The listing builds one solid part. Answer for the finished solid, in the listing's coordinates (mm). A direction names the side the tool comes from. Give positions to 0.01 mm unless a question says otherwise; leave off trailing zeros. Loops run counter-clockwise (first coordinate to the right, second up) from the corner with the lowest first, then second, coordinate; pieces in that order, holes last. Notation, with made-up numbers: (13, 59.5) - (20, 59.5) arc R24 cw to (20, 89.5) - close; hole circle Ø3 at (-10.75, -30.75). An arc over 180 degrees is marked (long way). Answer as CSV lines item,"result". Start each with the question number.
1) A cutting plane is placed at C-C (z = -11.5). Determine the outline of the cut face in (x, y), and give its area (3 significant figures).
2) A cutting plane is placed at D-D (x = 28). Determine the outline of the cut face in (y, z).
3) For a pull along Z with two mould halves and no side action, classify faces 3 (the face through (15.02, -0.02, 47.69)), 4 (the face through (18.377, 1.327, -36.344)), 5 (the face through (-1, -1.5, -1)) as pulls with the +Z half, pulls with the -Z half, needs draft (parallel to the pull), parting line crosses it, or undercut.
4) A cutting plane is placed at B-B (y = 0.4). Give the number of separate pieces and of enclosed holes in the cut face, and give its area (3 significant figures).
5) For faces 1 (the face through (19.672, 0.021, 21.94)), 2 (the face through (19.13, 0.99, 37.02)), determine the directions among +Z, -Z, +X, -X, +Y, -Y from which every point of the face is accessible in a straight line to the end or side of a thin tool.
6) Find the intervals of material crossed by line 1 along Z through (x, y) = (12, 1.1); line 2 along X through (y, z) = (1.2, 36.5); line 3 along Z through (x, y) = (4.5, -0.2), in increasing order.
7) A cutting plane is placed at A-A (x = 0). Determine the outline of the cut face in (y, z), and give its area (3 significant figures).
8) A flat-ended cylindrical pin translates along its axis: pin 1 (4 mm diameter, centred on x = -17.01, z = -38.13, fed in from +Y). Find the tip coordinate at first contact, or state that the pin passes through.
```python
from build123d import *

# Parameters (mm, degrees)
A_BASE_T_START                                = -1.5
A_BASE_T_OUTLINE_R                            = 47
A_BASE_T_OUTLINE_R_2                          = 1
A_BASE_T_DEPTH                                = 3
BASE_PULLEY_CUTOUT_DEPTH                      = 67.535704701
OUTER_START                                   = -3
SKETCH2_R                                     = 50
SKETCH2_R_2                                   = 47
OUTER_RING_DEPTH                              = 3
PATCHING_START                                = -3
SKETCH3_R                                     = 1
PATCHING_DEPTH                                = 3
CSK_FOR_8_FLAT_HEAD_SOCKET_CAP_SCREW1_A_COUNT = 2
CSK_FOR_8_FLAT_HEAD_SOCKET_CAP_SCREW1_A_PITCH = 34.018518517
CSK_FOR_8_FLAT_HEAD_SOCKET_CAP_SCRE_2_COUNT   = 2
CSK_FOR_8_FLAT_HEAD_SOCKET_CAP_SCRE_2_PITCH   = 83.5
CSK_FOR_8_FLAT_HEAD_SOCKET_CAP_SCRE_3_COUNT   = 2
CSK_FOR_8_FLAT_HEAD_SOCKET_CAP_SCRE_3_PITCH   = 76.256084334


# Read off the part's stored shape, not the designer's step: a_base_t
with BuildPart() as part:
    # a_base_t outline → a_base_t (new body)
    with BuildSketch(Plane(origin=(0, 0, 0), x_dir=(1, 0, 0), z_dir=(0, 1, 0)).offset(A_BASE_T_START)):
        Circle(A_BASE_T_OUTLINE_R)
        with Locations((-17.009259258, -38.128042167)):
            Circle(A_BASE_T_OUTLINE_R_2, mode=Mode.SUBTRACT)
        with Locations((-9.166666665, -28.284271247)):
            Circle(A_BASE_T_OUTLINE_R_2, mode=Mode.SUBTRACT)
        with Locations((17.009259258, -38.128042167)):
            Circle(A_BASE_T_OUTLINE_R_2, mode=Mode.SUBTRACT)
        with Locations((27.5, -28.284271247)):
            Circle(A_BASE_T_OUTLINE_R_2, mode=Mode.SUBTRACT)
        with Locations((-27.5, 28.284271247)):
            Circle(A_BASE_T_OUTLINE_R_2, mode=Mode.SUBTRACT)
        with Locations((-17.009259258, 38.128042167)):
            Circle(A_BASE_T_OUTLINE_R_2, mode=Mode.SUBTRACT)
        with Locations((9.166666665, 28.284271247)):
            Circle(A_BASE_T_OUTLINE_R_2, mode=Mode.SUBTRACT)
        with Locations((17.009259258, 38.128042167)):
            Circle(A_BASE_T_OUTLINE_R_2, mode=Mode.SUBTRACT)
    extrude(amount=A_BASE_T_DEPTH)

    # Sketch1 → Base Pulley Cutout (cut, through all)
    with BuildSketch(Plane(origin=(0, 1.5, 0), x_dir=(1, 0, 0), z_dir=(0, 1, 0))):
        Polygon((8.337949793, -17.780503881), (17.375186195, -14.85162044), (15.217061554, -8.192604143), (6.179825152, -11.121487584), align=None)
        Polygon((9.571163873, -21.58565605), (18.608400275, -18.656772609), (20.766524916, -25.315788906), (11.729288514, -28.244672346), align=None)
        Polygon((7.518722658, 15.561058274), (-1.518513745, 12.632174833), (-3.676638385, 19.291191129), (5.360598017, 22.22007457), align=None)
        Polygon((-4.909852466, 23.096343299), (4.127383937, 26.025226739), (1.969259296, 32.684243036), (-7.067977106, 29.755359595), align=None)
    extrude(amount=-BASE_PULLEY_CUTOUT_DEPTH, mode=Mode.SUBTRACT)

    # Sketch2 → Outer Ring (add)
    with BuildSketch(Plane(origin=(0, 1.5, 0), x_dir=(1, 0, 0), z_dir=(0, 1, 0)).offset(OUTER_START)):
        with Locations(Location((0, 0, 0), (0, 0, 270))):
            Circle(SKETCH2_R)
        Circle(SKETCH2_R_2, mode=Mode.SUBTRACT)
    extrude(amount=OUTER_RING_DEPTH)

    # Sketch3 → Patching (add)
    with BuildSketch(Plane(origin=(0, 1.5, 0), x_dir=(1, 0, 0), z_dir=(0, 1, 0)).offset(PATCHING_START)):
        with Locations((-9.166666665, -28.284271247)):
            Circle(SKETCH3_R)
        with Locations((-27.5, 28.284271247)):
            Circle(SKETCH3_R)
        with Locations((9.166666665, 28.284271247)):
            Circle(SKETCH3_R)
        with Locations((27.5, -28.284271247)):
            Circle(SKETCH3_R)
    extrude(amount=PATCHING_DEPTH)

    # Sketch6 → CSK for #8 Flat Head Socket Cap Screw1 (revolve, cut)
    with BuildSketch(Plane(origin=(17.009259258, -1.5, 38.128042167), x_dir=(0, 0, -1), z_dir=(1, 0, 0))):
        Polygon((0, 0), (0, 3), (2.2479, 3), (2.2479, 2.658961536), (4.5593, 0), align=None)
    csk_for_8_flat_head_socket_cap_screw1 = revolve(axis=Axis((17.009259258, -7.85, 38.128042167), (0, 1, 0)), mode=Mode.SUBTRACT)

    # CSK for #8 Flat Head Socket Cap Screw1 a: CSK for #8 Flat Head Socket Cap Screw1 ×2
    with Locations(*[(-i * CSK_FOR_8_FLAT_HEAD_SOCKET_CAP_SCREW1_A_PITCH, 0, 0) for i in range(1, CSK_FOR_8_FLAT_HEAD_SOCKET_CAP_SCREW1_A_COUNT)]):
        add(csk_for_8_flat_head_socket_cap_screw1, mode=Mode.SUBTRACT)

    # CSK for _8 Flat Head Socket Cap Scre 2: CSK for #8 Flat Head Socket Cap Screw1 ×2
    with Locations(*[Vector(-0.40740740738888753, 0, -0.9132465189666288) * (i * CSK_FOR_8_FLAT_HEAD_SOCKET_CAP_SCRE_2_PITCH) for i in range(1, CSK_FOR_8_FLAT_HEAD_SOCKET_CAP_SCRE_2_COUNT)]):
        add(csk_for_8_flat_head_socket_cap_screw1, mode=Mode.SUBTRACT)

    # CSK for _8 Flat Head Socket Cap Scre 3: CSK for #8 Flat Head Socket Cap Screw1 ×2
    with Locations(*[(0, 0, -i * CSK_FOR_8_FLAT_HEAD_SOCKET_CAP_SCRE_3_PITCH) for i in range(1, CSK_FOR_8_FLAT_HEAD_SOCKET_CAP_SCRE_3_COUNT)]):
        add(csk_for_8_flat_head_socket_cap_screw1, mode=Mode.SUBTRACT)


solid = part.part
```
Ans:
1,outline,"(-48.66, -1.5) - (48.66, -1.5) - (48.66, 1.5) - (-48.66, 1.5) - close"
1,area,"292 mm2"
2,outline,"(-1.5, -41.42) - (1.5, -41.42) - (1.5, 41.42) - (-1.5, 41.42) - close"
3,face 3,"parting line crosses it"
3,face 4,"undercut"
3,face 5,"needs draft"
4,separate pieces,"1"
4,enclosed holes,"8"
4,area,"7,480 mm2"
5,face 1,"+Y, -Y"
5,face 2,"-Y"
6,line 1,"-48.54 to 9.24, 16.59 to 20.8, 28.16 to 48.54"
6,line 2,"-34.17 to -18.56, -15.46 to 15.46, 18.56 to 34.17"
6,line 3,"-49.8 to -21.94, -14.58 to 49.8"
7,outline,"(-1.5, -50) - (1.5, -50) - (1.5, -32.05) - (-1.5, -32.05) - close; (-1.5, -24.69) - (1.5, -24.69) - (1.5, -20.48) - (-1.5, -20.48) - close; (-1.5, -13.12) - (1.5, -13.12) - (1.5, 50) - (-1.5, 50) - close"
7,area,"256 mm2"
8,pin 1,"through"
